from build123d import *

# Parameters (mm, degrees)
BOSS_EXTRUDE1_DEPTH     = 15.875
CUT_EXTRUDE1_DEPTH      = 59.973007597
CUT_EXTRUDE1_DEPTH_BACK = 59.973007597
SKETCH2_R               = 3.429


with BuildPart() as part:
    # Sketch1 → Boss-Extrude1 (new, symmetric)
    with BuildSketch(Plane(origin=(0, 0, 0), x_dir=(0, 0, -1), z_dir=(1, 0, 0))):
        Polygon((0, 0), (19.05, 0), (19.05, 25.4), (31.75, 25.4), (50.8, 25.4), (50.8, 30.48), (31.75, 30.48), (12.7, 30.48), (12.7, 5.08), (0, 5.08), align=None)
    extrude(amount=BOSS_EXTRUDE1_DEPTH, both=True)

    # Sketch2 → Cut-Extrude1 (cut, two sides: drawn at the far end of the back side and taken through both)
    with BuildSketch(Plane(origin=(0, 5.08, 0), x_dir=(1, 0, 0), z_dir=(0, 1, 0)).offset(-CUT_EXTRUDE1_DEPTH_BACK)):
        with Locations(Location((-6.35, 6.35, 0), (0, 0, 270))):
            Circle(SKETCH2_R)
        with Locations(Location((6.35, 6.35, 0), (0, 0, 270))):
            Circle(SKETCH2_R)
        with BuildLine():
            Line((-2.921, 44.45), (-2.921, 25.4))
            ThreePointArc((-2.921, 25.4), (-6.35, 21.971), (-9.779, 25.4))
            Line((-9.779, 25.4), (-9.779, 44.45))
            ThreePointArc((-9.779, 44.45), (-6.35, 47.879), (-2.921, 44.45))
        make_face()
        with BuildLine():
            Line((9.779, 44.45), (9.779, 25.4))
            ThreePointArc((9.779, 25.4), (6.35, 21.971), (2.921, 25.4))
            Line((2.921, 25.4), (2.921, 44.45))
            ThreePointArc((2.921, 44.45), (6.35, 47.879), (9.779, 44.45))
        make_face()
    extrude(amount=CUT_EXTRUDE1_DEPTH + CUT_EXTRUDE1_DEPTH_BACK, mode=Mode.SUBTRACT)


solid = part.part
Work out the finished part from the listing and answer in its coordinate system (mm). A direction names the side the tool comes from. Give positions to 0.01 mm unless a question says otherwise; leave off trailing zeros. Loops run counter-clockwise (first coordinate to the right, second up) from the corner with the lowest first, then second, coordinate; pieces in that order, holes last. Notation, with made-up numbers: M 30.5,18.5 L 89.5,18.5 A18 cw 89.5,37.5 Z; hole C 85,17 d10. An arc over 180 degrees is marked long. Use CSV: the item, a comma, the result in double quotes.
1) Which of the six approach directions +Z, -Z, +X, -X, +Y, -Y give full straight-line access (tool end or side, diameter ignored) to faces 4 (the flat face through (0, 18, -12.7)), 5 (the cylindrical face through (6.43, 27.9, -21.97)), 6 (the flat face through (0, 13, -19.05))?
Answer:
face 4,"+Z, +X, -X, +Y"
face 5,"+Y, -Y"
face 6,"-Z, +X, -X, -Y"
2) Find section A-A on x = -6.35. Write down the section's boundary in (y, z).
Answer:
outline,"M 0,-19.05 L 25.4,-19.05 L 25.4,-21.97 L 30.48,-21.97 L 30.48,-12.7 L 5.08,-12.7 L 5.08,-9.78 L 0,-9.78 Z; M 0,-2.92 L 5.08,-2.92 L 5.08,0 L 0,0 Z; M 25.4,-50.8 L 30.48,-50.8 L 30.48,-47.88 L 25.4,-47.88 Z"
3) Consider L1, parallel to X at y = 1.7, z = -6.35 (3 decimals); L2, parallel to Z at x = 6.35, y = 3.9; L3, parallel to Y at x = 2, z = -45. Determine where each line is inside the solid, lowest interval first.
Answer:
L1,"-15.875 to -9.779, -2.921 to 2.921, 9.779 to 15.875"
L2,"-19.05 to -9.78, -2.92 to 0"
L3,"25.4 to 30.48"
4) Find section C-C on y = 4. Write down the section's boundary in (x, z) (3 decimals).
Answer:
outline,"M -15.875,-19.05 L 15.875,-19.05 L 15.875,0 L -15.875,0 Z; hole C -6.35,-6.35 d6.858; hole C 6.35,-6.35 d6.858"
5) Find section D-D on z = -24. Write down the section's boundary in (x, y) (3 decimals).
Answer:
outline,"M -15.875,25.4 L -9.48,25.4 L -9.48,30.48 L -15.875,30.48 Z; M -3.22,25.4 L 3.22,25.4 L 3.22,30.48 L -3.22,30.48 Z; M 9.48,25.4 L 15.875,25.4 L 15.875,30.48 L 9.48,30.48 Z"
6) Find section B-B on z = -6.35. Write down the section's boundary in (x, y) (3 decimals), plus the area to 3 significant figures.
Answer:
outline,"M -15.875,0 L -9.779,0 L -9.779,5.08 L -15.875,5.08 Z; M -2.921,0 L 2.921,0 L 2.921,5.08 L -2.921,5.08 Z; M 9.779,0 L 15.875,0 L 15.875,5.08 L 9.779,5.08 Z"
area,"91.6 mm^2"
7) Given P1, Ø5.5, axis at x = -6.35, z = -6.35, coming from the +Y side; P2, Ø6, axis at x = -6.5, y = 13, coming from the -Z side; P3, Ø1, axis at x = 10.5, z = -31, coming from the -Y side; P4, Ø3, axis at x = -9.5, y = 21, coming from the +Z side, each flat-ended and moving along its own axis, determine where each tip first touches the part or whether it passes through.
Answer:
P1,"through"
P2,"z = -19.05"
P3,"y = 25.4"
P4,"z = -12.7"
8) Determine the mould class of faces 1 (the flat face through (0, 5.08, -6)), 2 (the cylindrical face through (-6.27, 27.9, -21.97)), 3 (the flat face through (-15.875, 20, -18)) for opening direction X: released by +X, released by -X, zero draft, split by the parting line, or undercut.
Answer:
face 1,"zero draft"
face 2,"undercut"
face 3,"released by -X"
